Geometry check sheet. Reference: the model listing, model coordinates, mm. Face numbers are marked on the shaded views. A direction names the side the tool comes from. Round coordinates to 2 decimals unless told otherwise and drop trailing zeros. Write each loop counter-clockwise with the first axis right and the second up, starting at its lowest first coordinate (ties: lowest second). Pieces come first, ordered by that corner, then holes. Notation, with made-up numbers: (4, -19.75) - (55, -19.75) arc R12 cw to (55, -10.75) - close; hole circle Ø8 at (70, -39.75). An arc over 180 degrees is marked (long way). Return JSON: item names as keys, results as strings.
```python
from build123d import *

# Parameters (mm, degrees)
F3_R     = 18.2754285366
F4_DEPTH = 251
F5_R     = 16.060733565
F6_DEPTH = 127.001


# Not quite as in the source:
# - an extrude ends at something that could not be found from the text; its depth is read off the source's solid


with BuildPart() as f1:
    # F0 (on Front) → F1 (revolve)
    with BuildSketch(Plane.XZ):
        Polygon((0, 127), (0, 0), (19.05, 0), (19.05, 12.7), (50.8, 12.7), (50.8, 25.4), (19.05, 25.4), (19.05, 38.1), (50.8, 38.1), (50.8, 50.8), (19.05, 50.8), (19.05, 63.5), (50.8, 63.5), (50.8, 76.2), (19.05, 76.2), (19.05, 88.9), (50.8, 88.9), (50.8, 101.6), (19.05, 101.6), (19.05, 114.3), (50.8, 114.3), (50.8, 127), align=None)
    revolve(axis=Axis((0, 0, 63.5), (0, 0, 1)))

    # F3 (on face) → F4 (cut, through all)
    with BuildSketch(Plane.XY.offset(127)):
        Circle(F3_R)
    extrude(amount=F4_DEPTH, mode=Mode.SUBTRACT)

    # F5 (on face) → F6 (cut, through all)
    with BuildSketch(Plane.XY.offset(127)):
        Circle(F5_R)
    extrude(amount=-F6_DEPTH, mode=Mode.SUBTRACT)


solid = f1.part
```
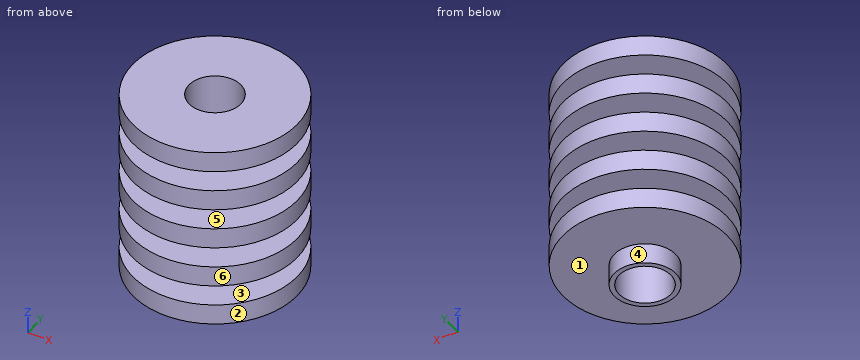
(1) Gauge pin test, flat ends, axial feed: pin 1 (4 mm diameter, centred on x = -27, z = 93.5, fed in from -Y); pin 2 (3 mm diameter, centred on y = 13.5, z = 83, fed in from +X); pin 3 (5 mm diameter, centred on x = 10.5, y = 19, fed in from -Z); pin 4 (1.5 mm diameter, centred on y = 28.5, z = 104, fed in from -X). Record the tip position at first contact, or that the pin passes through.
Response values:
{"pin 1": "stops at y = -44.22", "pin 2": "stops at x = 14.8", "pin 3": "stops at z = 12.7", "pin 4": "passes through"}
(2) Release check for a two-part mould opening along Z. For the marked faces 1, 2 and 3 record: pulls with the +Z half, pulls with the -Z half, needs draft (parallel to the pull), parting line crosses it, or undercut.
Response values:
{"face 1": "pulls with the -Z half", "face 2": "needs draft", "face 3": "undercut"}
(3) Material ranges on line 1 along Z through (x, y) = (17, 45); line 2 along Y through (x, z) = (0, 82); line 3 along Y through (x, z) = (0, 90.5), recorded low to high. Write a range as [from, to].
Response values:
{"line 1": "z = [12.7, 25.4], [38.1, 50.8], [63.5, 76.2], [88.9, 101.6], [114.3, 127]", "line 2": "y = [-19.05, -16.06], [16.06, 19.05]", "line 3": "y = [-50.8, -16.06], [16.06, 50.8]"}
(4) Section check A-A, the plane x = -39.5. Enter the section's corners in (y, z).
Response values:
{"outline": "(-31.94, 12.7) - (31.94, 12.7) - (31.94, 25.4) - (-31.94, 25.4) - close; (-31.94, 38.1) - (31.94, 38.1) - (31.94, 50.8) - (-31.94, 50.8) - close; (-31.94, 63.5) - (31.94, 63.5) - (31.94, 76.2) - (-31.94, 76.2) - close; (-31.94, 88.9) - (31.94, 88.9) - (31.94, 101.6) - (-31.94, 101.6) - close; (-31.94, 114.3) - (31.94, 114.3) - (31.94, 127) - (-31.94, 127) - close"}
(5) Access from +Z, -Z, +X, -X, +Y, -Y to the whole of each face (thin tool, end or side, straight path). Record for the marked faces 4, 5 and 6.
Response values:
{"face 4": "-Z", "face 5": "none", "face 6": "+Z, -Z"}
